Input: dimensioned drawing with shaded views. Units: mm. Origin: part minimum x, y, z. A direction names the side the tool comes from. Round coordinates to 2 decimals unless told otherwise and drop trailing zeros. Loops run counter-clockwise (first coordinate to the right, second up) from the corner with the lowest first, then second, coordinate; pieces in that order, holes last. Notation, with made-up numbers: (85, 10.25) - (141, 10.25) arc R13 cw to (141, 30.25) - close; hole circle Ø11 at (-8, 81.25). An arc over 180 degrees is marked (long way). One line per question, with ' | ' between items. Start each with the question number.
Item 1: Section A-A, the plane z = 3. Give the number of separate pieces and of enclosed holes in the cut face, plus the area to 3 significant figures.
Item 2: Material intervals for line 1 along Y through (x, z) = (71, 17); line 2 along X through (y, z) = (11.5, 8) (1 decimal); line 3 along Z through (x, y) = (23, 15), sorted ascending.
Item 3: Section D-D, the plane y = 28. Return loops of the section in (x, z).
Item 4: Set-up query: the marked faces 4 and 5. Return all of +Z, -Z, +X, -X, +Y, -Y with unobstructed straight access to the full face (end or side cutting, diameter ignored); none if empty.
Item 5: First-contact query: pin 1 (3 mm diameter, centred on y = 58.5, z = 13.5, fed in from +X); pin 2 (10 mm diameter, centred on y = 27, z = 14, fed in from +X); pin 3 (6 mm diameter, centred on y = 43.5, z = 27, fed in from +X); pin 4 (13 mm diameter, centred on x = 21.77, y = 30, fed in from +Z). Flat tips, straight axial feed; report the tip coordinate or a pass-through.
Item 6: Draft query along X for the marked faces 1, 2 and 3. Return one class per face: pulls with the +X half, pulls with the -X half, needs draft (parallel to the pull), parting line crosses it, or undercut.
Item 7: Section C-C, the plane x = 58.5. Return loops of the section in (y, z), plus the area to 3 significant figures.
Item 8: Section B-B, the plane y = 14. Return loops of the section in (x, z), plus the area to 3 significant figures.
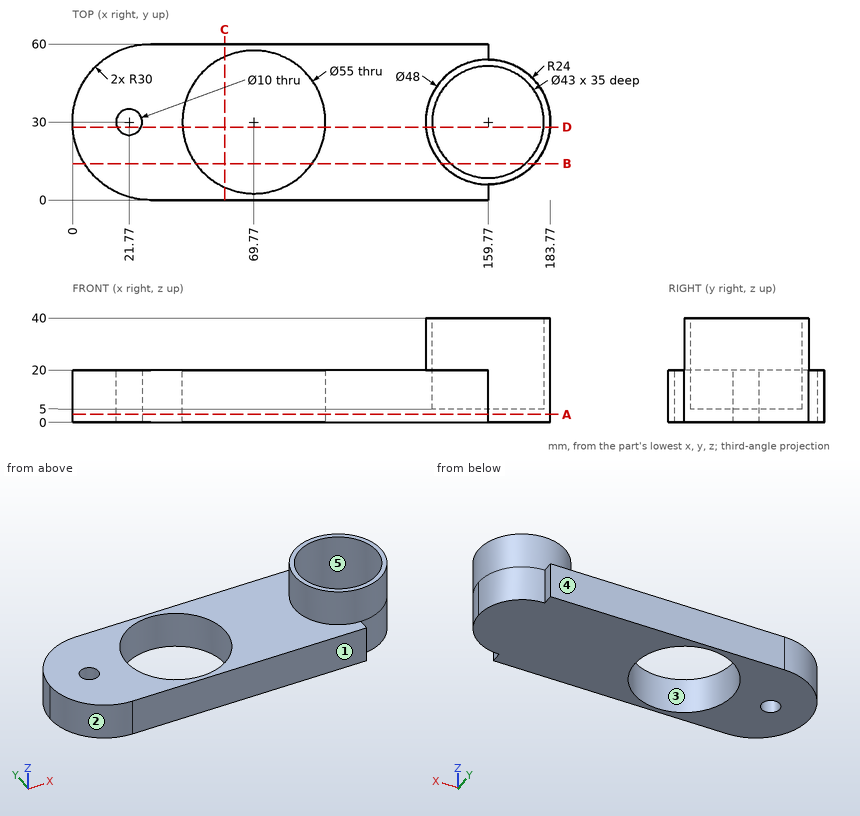
Return value:
1) separate pieces: 1 | enclosed holes: 2 | area: 7,650 mm2
2) line 1: 0 to 2.53, 57.47 to 60 | line 2: 6.4 to 49.4, 90.1 to 148.8, 170.7 to 175.1 | line 3: 0 to 20
3) outline: (0.07, 0) - (17.19, 0) - (17.19, 20) - (0.07, 20) - close; (26.35, 0) - (42.34, 0) - (42.34, 20) - (26.35, 20) - close; (97.2, 0) - (183.69, 0) - (183.69, 40) - (181.18, 40) - (181.18, 5) - (138.36, 5) - (138.36, 40) - (135.85, 40) - (135.85, 20) - (97.2, 20) - close
4) face 4: +Z, -Z, +X, -X, +Y | face 5: +Z
5) pin 1: x = 159.77 | pin 2: x = 183.77 | pin 3: x = 181.35 | pin 4: z = 20
6) face 1: needs draft | face 2: pulls with the -X half | face 3: undercut
7) outline: (0, 0) - (4.92, 0) - (4.92, 20) - (0, 20) - close; (55.08, 0) - (60, 0) - (60, 20) - (55.08, 20) - close | area: 197 mm2
8) outline: (4.62, 0) - (47.4, 0) - (47.4, 20) - (4.62, 20) - close; (92.14, 0) - (177.66, 0) - (177.66, 40) - (174.13, 40) - (174.13, 5) - (145.41, 5) - (145.41, 40) - (141.88, 40) - (141.88, 20) - (92.14, 20) - close | area: 2,280 mm2
